Here's how the part is built. I have some questions about the finished solid (model axes, mm). Face numbers are marked on the shaded views. A direction names the side the tool comes from. Give positions to 0.01 mm unless a question says otherwise; leave off trailing zeros. Order: outer loops, then holes, each group sorted by start corner. A loop starts at its lowest first (then second) coordinate and runs counter-clockwise, first axis right, second up.
from build123d import *

# Parameters (mm, degrees)
F1_DEPTH = 4
F3_DEPTH = 6
F4_R     = 5
F5_DEPTH = 6
F7_DEPTH = 10.001


with BuildPart() as f1:
    # F0 (on Top) → F1 (new body)
    with BuildSketch(Plane.XY):
        with BuildLine():
            Line((56.2, 7.846018), (25.42, 32.168674))
            ThreePointArc((25.42, 32.168674), (-41, 0), (25.42, -32.168674))
            Line((25.42, -32.168674), (56.2, -7.846018))
            ThreePointArc((56.2, -7.846018), (60, 0), (56.2, 7.846018))
        make_face()
    extrude(amount=F1_DEPTH)

    # F2 (on face) → F3 (join)
    with BuildSketch(Plane.XY.offset(4)):
        with BuildLine():
            ThreePointArc((25.618741, -23.847015), (19.7, 0), (25.618741, 23.847015))
            ThreePointArc((25.618741, 23.847015), (-35, 0), (25.618741, -23.847015))
        make_face()
    extrude(amount=F3_DEPTH)

    # F4 (on face) → F5 (join)
    with BuildSketch(Plane.XY.offset(4)):
        with Locations((50, 0)):
            Circle(F4_R)
    extrude(amount=F5_DEPTH)

    # F6 (on face) → F7 (cut, through all)
    with BuildSketch(Plane.XY.offset(10)):
        with BuildLine():
            Line((3, 4), (-3, 4))
            ThreePointArc((-3, 4), (-5, 0), (-3, -4))
            Line((-3, -4), (3, -4))
            ThreePointArc((3, -4), (5, 0), (3, 4))
        make_face()
    extrude(amount=-F7_DEPTH, mode=Mode.SUBTRACT)


solid = f1.part
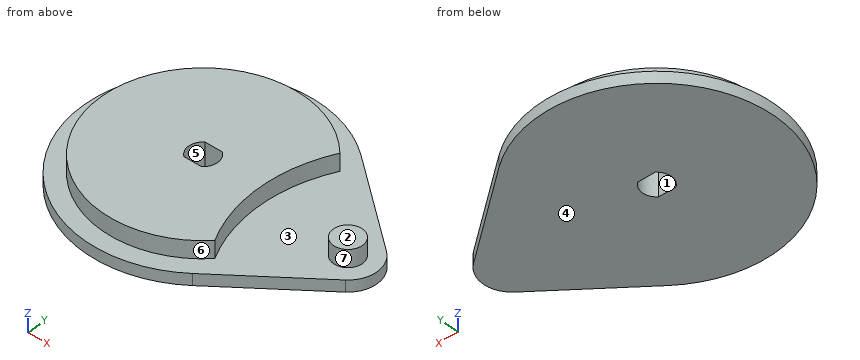
Q1. If we section it at C-C on x = -20.5: List the corners of the cut face in (y, z) for me.
Filled sheet:
outline: (-35.51, 0) - (35.51, 0) - (35.51, 4) - (28.37, 4) - (28.37, 10) - (-28.37, 10) - (-28.37, 4) - (-35.51, 4) - close
Q2. If we section it at A-A on x = 0: List the corners of the cut face in (y, z) for me, plus the area to 3 significant figures.
Filled sheet:
outline: (-41, 0) - (-4, 0) - (-4, 10) - (-35, 10) - (-35, 4) - (-41, 4) - close; (4, 0) - (41, 0) - (41, 4) - (35, 4) - (35, 10) - (4, 10) - close
area: 668 mm2
Q3. If we section it at D-D on y = -9: List the corners of the cut face in (x, z) for me, plus the area to 3 significant figures.
Filled sheet:
outline: (-40, 0) - (54.74, 0) - (54.74, 4) - (20.5, 4) - (20.5, 10) - (-33.82, 10) - (-33.82, 4) - (-40, 4) - close
area: 705 mm2
Q4. If we section it at B-B on y = 0: List the corners of the cut face in (x, z) for me, plus the area to 3 significant figures.
Filled sheet:
outline: (-41, 0) - (-5, 0) - (-5, 10) - (-35, 10) - (-35, 4) - (-41, 4) - close; (5, 0) - (60, 0) - (60, 4) - (55, 4) - (55, 10) - (45, 10) - (45, 4) - (19.7, 4) - (19.7, 10) - (5, 10) - close
area: 692 mm2
Q5. I'm going to push flat-ended pins straight in: P1, Ø1, axis at x = 13.5, z = 5.5, coming from the -Y side; P2, Ø2, axis at x = 18, z = 7, coming from the +Y side; P3, Ø5, axis at x = -2.5, z = 3.5, coming from the +Y side. Where does each tip first touch, or does it pass through?
Filled sheet:
P1: stops at y = -32.5
P2: stops at y = 30.59
P3: stops at y = 41
Q6. I need wall thicknesses on L1, parallel to X at y = 3, z = 8.75; L2, parallel to Y at x = 50, z = 7.25; L3, parallel to Z at x = 28, y = -6.5. Which ranges of each line are inside material? Lowest first, please.
Filled sheet:
L1: x = -34.87 to -4, 4 to 19.79, 46 to 54
L2: y = -5 to 5
L3: z = 0 to 4
Q7. Thinking about a two-plate mould opening in X: for the marked faces 4, 5, 6 and 7, which applies, released by +X, released by -X, zero draft, split by the parting line, or undercut?
Filled sheet:
face 4: zero draft
face 5: undercut
face 6: split by the parting line
face 7: undercut
Q8. For the marked faces 1, 2 and 3, which set-ups out of +Z, -Z, +X, -X, +Y, -Y let a thin tool reach every point of the face, with its end or its side?
Filled sheet:
face 1: +Z, -Z
face 2: +Z, +X, -X, +Y, -Y
face 3: +Z
